Model file for the job. Use its own axes, mm. A direction names the side the tool comes from. Coordinates: 2 decimals unless noted, no trailing zeros. Order: outer loops, then holes, each group sorted by start corner. A loop starts at its lowest first (then second) coordinate and runs counter-clockwise, first axis right, second up.
from build123d import *

# Parameters (mm, degrees)
SKETCH011_W     = 3
SKETCH011_H     = 9
SKETCH012_W     = 3
SKETCH012_H     = 3
SKETCH_W        = 70
SKETCH_H        = 50
PAD_DEPTH       = 30
POCKET_DEPTH    = 20
SKETCH002_W     = 3
SKETCH002_H     = 30
PAD001_DEPTH    = 19
SKETCH003_W     = 3
SKETCH003_H     = 26
PAD002_DEPTH    = 19
SKETCH004_W     = 2
SKETCH004_H     = 29
PAD003_DEPTH    = 1
SKETCH005_W     = 2
SKETCH005_H     = 25
PAD004_DEPTH    = 1
FILLET_R        = 1.9
SKETCH006_R     = 2.5
POCKET001_DEPTH = 12
SKETCH007_W     = 2
SKETCH007_H     = 2
SKETCH009_W     = 80
SKETCH009_H     = 80
SKETCH009_W_2   = 56
SKETCH009_H_2   = 36
POCKET002_DEPTH = 40
SKETCH010_W     = 80
SKETCH010_H     = 80
POCKET003_DEPTH = 7
SKETCH013_W     = 2
SKETCH013_H     = 2
POCKET004_DEPTH = 5
FILLET001_R     = 2
PAD005_DEPTH    = 19


with BuildPart() as loft_body:
    # Sketch011 (on Face42 of Pocket003) → Loft section 0
    with BuildSketch(Plane(origin=(0, 13, 0), x_dir=(-1, 0, 0), z_dir=(0, 1, 0))):
        with Locations((-13.5, 10.5)):
            Rectangle(SKETCH011_W, SKETCH011_H)
    # Sketch012 (on Face36 of Pocket003) → Loft section 1
    with BuildSketch(Plane(origin=(0, 18, 0), x_dir=(-1, 0, 0), z_dir=(0, 1, 0))):
        with Locations((-13.5, 10.5)):
            Rectangle(SKETCH012_W, SKETCH012_H)
    loft()


with BuildPart() as body001:
    # Sketch → Pad (new body)
    with BuildSketch(Plane.XY):
        Rectangle(SKETCH_W, SKETCH_H)
    extrude(amount=PAD_DEPTH)

    # Sketch001 (on Face5 of Pad) → Pocket (cut)
    with BuildSketch(Plane(origin=(0, 0, 0), x_dir=(1, 0, 0), z_dir=(0, 0, -1))):
        Polygon((-35, 15), (-25, 15), (-25, 25), (25, 25), (25, 15), (35, 15), (35, -15), (25, -15), (25, -25), (-25, -25), (-25, -15), (-35, -15), align=None)
    extrude(amount=-POCKET_DEPTH, mode=Mode.SUBTRACT)

    # Sketch002 (on Face4 of Pocket) → Pad001 (join)
    with BuildSketch(Plane(origin=(0, 0, 20), x_dir=(1, 0, 0), z_dir=(0, 0, -1))):
        with Locations((-18.5, 0)):
            Rectangle(SKETCH002_W, SKETCH002_H)
        with Locations((18.5, 0)):
            Rectangle(SKETCH002_W, SKETCH002_H)
    extrude(amount=PAD001_DEPTH)

    # Sketch003 (on Face4 of Pad001) → Pad002 (join)
    with BuildSketch(Plane(origin=(0, 0, 20), x_dir=(1, 0, 0), z_dir=(0, 0, -1))):
        with Locations((13.5, 0)):
            Rectangle(SKETCH003_W, SKETCH003_H)
        with Locations((-13.5, 0)):
            Rectangle(SKETCH003_W, SKETCH003_H)
    extrude(amount=PAD002_DEPTH)

    # Sketch004 (on Face36 of Pad002) → Pad003 (join)
    with BuildSketch(Plane(origin=(0, 0, 1), x_dir=(1, 0, 0), z_dir=(0, 0, -1))):
        with Locations((18.5, 0)):
            Rectangle(SKETCH004_W, SKETCH004_H)
        with Locations((-18.5, 0)):
            Rectangle(SKETCH004_W, SKETCH004_H)
    extrude(amount=PAD003_DEPTH)

    # Sketch005 (on Face37 of Pad003) → Pad004 (join)
    with BuildSketch(Plane(origin=(0, 0, 1), x_dir=(1, 0, 0), z_dir=(0, 0, -1))):
        with Locations((-13.5, 0)):
            Rectangle(SKETCH005_W, SKETCH005_H)
        with Locations((13.5, 0)):
            Rectangle(SKETCH005_W, SKETCH005_H)
    extrude(amount=PAD004_DEPTH)

    # Fillet
    fillet_edges = [body001.edges().sort_by_distance(p)[0] for p in [
        (-19.5, 14.5, 0.5),
        (-14.5, 12.5, 0.5),
        (-19.5, -14.5, 0.5),
        (-14.5, -12.5, 0.5),
        (19.5, 14.5, 0.5),
        (14.5, 12.5, 0.5),
        (14.5, -12.5, 0.5),
        (19.5, -14.5, 0.5),
    ]]
    fillet(fillet_edges, radius=FILLET_R)

    # Sketch006 (on Face13 of Fillet) → Pocket001 (cut)
    with BuildSketch(Plane(origin=(0, 0, 20), x_dir=(1, 0, 0), z_dir=(0, 0, -1))):
        Circle(SKETCH006_R)
    extrude(amount=-POCKET001_DEPTH, mode=Mode.SUBTRACT)

    # Sketch007 (on Face13 of Pocket001) → Revolution (revolve)
    with BuildSketch(Plane(origin=(0, 0, 20), x_dir=(1, 0, 0), z_dir=(0, 0, -1))):
        with Locations((-7, 3)):
            Rectangle(SKETCH007_W, SKETCH007_H)
        with Locations((7, 3)):
            Rectangle(SKETCH007_W, SKETCH007_H)
    revolve(axis=Axis((-10, 0, 20), (1, 0, 0)))

    # Sketch009 (on Face49 of Revolution) → Pocket002 (cut)
    with BuildSketch(Plane.XY.offset(30)):
        Rectangle(SKETCH009_W, SKETCH009_H)
        Rectangle(SKETCH009_W_2, SKETCH009_H_2, mode=Mode.SUBTRACT)
    extrude(amount=-POCKET002_DEPTH, mode=Mode.SUBTRACT)

    # Sketch010 (on Face47 of Pocket002) → Pocket003 (cut)
    with BuildSketch(Plane.XY.offset(30)):
        Rectangle(SKETCH010_W, SKETCH010_H)
    extrude(amount=-POCKET003_DEPTH, mode=Mode.SUBTRACT)

    # Fusion: union Loft body
    add(loft_body.part)

    # Sketch013 (on Face56 of BaseFeature) → Pocket004 (cut)
    with BuildSketch(Plane(origin=(12, 0, 0), x_dir=(0, -1, 0), z_dir=(-1, 0, 0))):
        with Locations((-15.5, 10.5)):
            Rectangle(SKETCH013_W, SKETCH013_H)
    extrude(amount=-POCKET004_DEPTH, mode=Mode.SUBTRACT)

    # Fillet001
    fillet001_edges = [body001.edges().sort_by_distance(p)[0] for p in [
        (13.5, 18, 12),
        (13.5, 18, 9),
    ]]
    fillet(fillet001_edges, radius=FILLET001_R)

    # Sketch014 (on Face16 of Fillet001) → Pad005 (join)
    with BuildSketch(Plane(origin=(0, 0, 20), x_dir=(1, 0, 0), z_dir=(0, 0, -1))):
        Polygon((-17, 15), (-15, 13), (-15, -13), (-17, -15), align=None)
        Polygon((17, -15), (15, -13), (15, 13), (17, 15), align=None)
    extrude(amount=PAD005_DEPTH)


solid = body001.part
Q1. Cut at C-C, the plane y = -10. List the corners of the cut face in (x, z).
Established:
outline: (-28, 20) - (-20, 20) - (-20, 1) - (-19.5, 1) - (-19.5, 0) - (-17.5, 0) - (-17.5, 1) - (-14.5, 1) - (-14.5, 0) - (-12.5, 0) - (-12.5, 1) - (-12, 1) - (-12, 20) - (12, 20) - (12, 1) - (12.5, 1) - (12.5, 0) - (14.5, 0) - (14.5, 1) - (17.5, 1) - (17.5, 0) - (19.5, 0) - (19.5, 1) - (20, 1) - (20, 20) - (28, 20) - (28, 23) - (-28, 23) - close
Q2. Probe line 1 (X direction, y = 0, z = 22.2); line 2 (X direction, y = 3.5, z = 4.5); line 3 (Y direction, x = 0, z = 20.85). List the from-to ranges inside material, lowest first.
Established:
line 1: x = -28 to -2.5, 2.5 to 28
line 2: x = -20 to -12, 12 to 20
line 3: y = -18 to -2.5, 2.5 to 18
Q3. Drop flat-ended pins along their axis: P1, Ø6, axis at x = 16, z = 6.5, coming from the -Y side; P2, Ø0.5, axis at y = 2, z = 0.5, coming from the -X side; P3, Ø12, axis at y = 12.5, z = 10, coming from the -X side; P4, Ø0.9, axis at x = 13, z = 17.5, coming from the +Y side. Give the stop position or say it passes through.
Established:
P1: stops at y = -15
P2: stops at x = -19.5
P3: stops at x = -28
P4: stops at y = 13
Q4. Cut at A-A, the plane z = 7.5. Count the separate pieces of the cut face and the enclosed holes in it, plus the area to 4 significant figures.
Established:
separate pieces: 6
enclosed holes: 0
area: 491.5 mm2
Q5. Cut at B-B, the plane x = 0. List the corners of the cut face in (y, z).
Established:
outline: (-18, 20) - (-2.5, 20) - (-2.5, 23) - (-18, 23) - close; (2.5, 20) - (18, 20) - (18, 23) - (2.5, 23) - close
Q6. Mould opens along Y. For faces 6 (the face through (-0.54, 2.44, 21.48)), 7 (the face through (-18.929, -13.958, 0.493)), 8 (the face through (-7, 0, 16)) say: pulls with the +Y half, pulls with the -Y half, needs draft (parallel to the pull), parting line crosses it, or undercut.
Established:
face 6: undercut
face 7: pulls with the -Y half
face 8: parting line crosses it
Q7. Which spindle directions (+Z, -Z, +X, -X, +Y, -Y) get a long thin tool onto all of the face, cutting with end or side? Do faces 1 (the face through (-7, 0, 18)), 2 (the face through (16, -14, 11)), 3 (the face through (-8, -0.1, 17.5)), 4 (the face through (13.5, 15, 13.8)), 5 (the face through (-13.929, 11.958, 0.493)). Say none if no direction does.
Established:
face 1: none
face 2: -Z, -Y
face 3: -Z, +Y, -Y
face 4: +Y
face 5: -Z, +Y
